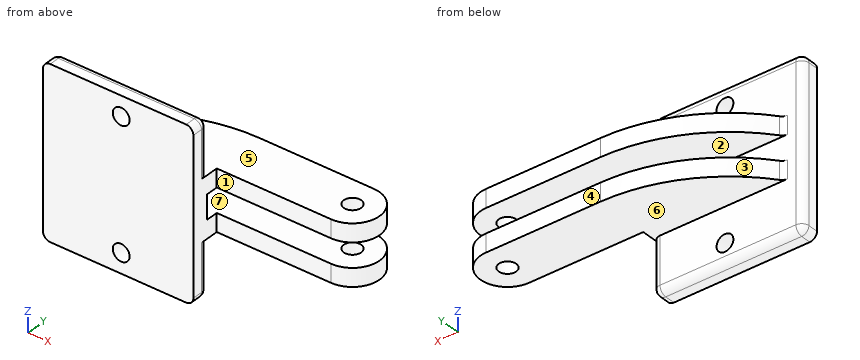
from build123d import *

# Parameters (mm, degrees)
SKETCH1_W           = 15.875
SKETCH1_H           = 17.78
SKETCH1_R           = 0.889
BOSS_EXTRUDE1_DEPTH = 1.8415
SKETCH2_R           = 0.92075
BOSS_EXTRUDE2_DEPTH = 3.175
SKETCH2_2_R         = 0.92075
CUT_EXTRUDE1_DEPTH  = 1.27
FILLET1_R           = 0.762


with BuildPart() as part:
    # Sketch1 → Boss-Extrude1 (new body)
    with BuildSketch(Plane(origin=(0, 0, 0), x_dir=(1, 0, 0), z_dir=(0, 1, 0))):
        Rectangle(SKETCH1_W, SKETCH1_H)
        with Locations((0.3175, 6.7945)):
            Circle(SKETCH1_R, mode=Mode.SUBTRACT)
        with Locations((0.3175, -6.7945)):
            Circle(SKETCH1_R, mode=Mode.SUBTRACT)
    extrude(amount=BOSS_EXTRUDE1_DEPTH)

    # Sketch2 → Boss-Extrude2 (add, symmetric)
    with BuildSketch(Plane.XY):
        with BuildLine():
            ThreePointArc((7.9375, 8.8265), (0.184776704, 6.981333441), (-5.9055, 1.8415))
            Line((-5.9055, 1.8415), (7.9375, 1.8415))
            Line((7.9375, 1.8415), (7.9375, 3.1115))
            Line((7.9375, 3.1115), (20.0025, 3.1115))
            ThreePointArc((20.0025, 3.1115), (22.86, 5.969), (20.0025, 8.8265))
            Line((20.0025, 8.8265), (7.9375, 8.8265))
        make_face()
        with Locations((20.0025, 5.969)):
            Circle(SKETCH2_R, mode=Mode.SUBTRACT)
    extrude(amount=BOSS_EXTRUDE2_DEPTH, both=True)

    # Sketch2<2> → Cut-Extrude1 (cut, symmetric)
    with BuildSketch(Plane.XY):
        with BuildLine():
            ThreePointArc((7.9375, 8.8265), (0.184776704, 6.981333441), (-5.9055, 1.8415))
            Line((-5.9055, 1.8415), (7.9375, 1.8415))
            Line((7.9375, 1.8415), (7.9375, 3.1115))
            Line((7.9375, 3.1115), (20.0025, 3.1115))
            ThreePointArc((20.0025, 3.1115), (22.86, 5.969), (20.0025, 8.8265))
            Line((20.0025, 8.8265), (7.9375, 8.8265))
        make_face()
        with Locations((20.0025, 5.969)):
            Circle(SKETCH2_2_R, mode=Mode.SUBTRACT)
    extrude(amount=CUT_EXTRUDE1_DEPTH, both=True, mode=Mode.SUBTRACT)

    # Fillet1
    fillet1_edges = [part.edges().sort_by_distance(p)[0] for p in [
        (7.9375, 1.8415, 6.0325),
        (0, 1.8415, -8.89),
        (7.9375, 1.8415, -6.0325),
        (-5.9055, 1.8415, 2.2225),
        (-5.9055, 1.8415, -2.2225),
        (-7.9375, 1.8415, 0),
        (-7.9375, 0.92075, -8.89),
        (7.9375, 0.92075, -8.89),
        (7.9375, 0.92075, 8.89),
        (-7.9375, 0.92075, 8.89),
        (0, 1.8415, 8.89),
    ]]
    fillet(fillet1_edges, radius=FILLET1_R)


solid = part.part
Verification items for the finished model (mm, model axes). Face numbers are marked on the shaded views. A direction names the side the tool comes from. Give positions to 0.01 mm unless a question says otherwise; leave off trailing zeros. Write each loop counter-clockwise with the first axis right and the second up, starting at its lowest first coordinate (ties: lowest second). Pieces come first, ordered by that corner, then holes. Notation, with made-up numbers: M -26.5,-20 L 6.5,-20 A22 cw 6.5,17 Z; hole C 27,80.5 d7. An arc over 180 degrees is marked long. Use CSV: the item, a comma, the result in double quotes.
1) Cross-section at C-C (z = -6.5). Enter the section's corners in (x, y).
Final values:
outline,"M -7.94,0 L -0.52,0 L -0.52,1.84 L -7.18,1.84 A0.76 ccw -7.94,1.08 Z; M 1.16,0 L 7.94,0 L 7.94,1.08 A0.76 ccw 7.18,1.84 L 1.16,1.84 Z"
2) Cross-section at D-D (z = 4.5). Enter the section's corners in (x, y), plus the area to 3 significant figures.
Final values:
outline,"M -7.94,0 L 7.94,0 L 7.94,1.08 A0.76 ccw 7.18,1.84 L -7.18,1.84 A0.76 ccw -7.94,1.08 Z"
area,"29.0 mm²"
3) Go/stop test with flat-tipped pins: pin 1 Ø2 at (x, z) = (0.32, 6.79) entering from +Y; pin 2 Ø7.5 at (x, z) = (1, 0.5) entering from +Y; pin 3 Ø2 at (x, y) = (-3.5, 5) entering from -Z (3 decimals). Record where each tip stops, or that it passes through.
Final values:
pin 1,"y = 1.84"
pin 2,"y = 8.51"
pin 3,"z = -3.175"
4) Access from +Z, -Z, +X, -X, +Y, -Y to the whole of each face (thin tool, end or side, straight path). Record for the marked faces 1, 2 and 3.
Final values:
face 1,"+Z, -Z, +X, -Y"
face 2,"+X, -X, +Y"
face 3,"+Z, -Z, -X, +Y"
5) Cross-section at A-A (x = 12.5). Enter the section's corners in (y, z) (1 decimal).
Final values:
outline,"M 3.1,-3.2 L 8.8,-3.2 L 8.8,-1.3 L 3.1,-1.3 Z; M 3.1,1.3 L 8.8,1.3 L 8.8,3.2 L 3.1,3.2 Z"
6) Material ranges on line 1 along Z through (x, y) = (18, 5.25) (3 decimals); line 2 along Y through (x, z) = (15, 2.5); line 3 along X through (y, z) = (0.5, 0.5), recorded low to high.
Final values:
line 1,"-3.175 to -1.27, 1.27 to 3.175"
line 2,"3.11 to 8.83"
line 3,"-7.94 to 7.94"
7) Cross-section at B-B (y = 4). Enter the section's corners in (x, z) (3 decimals), plus the area to 3 significant figures.
Final values:
outline,"M -4.014,-3.175 L 22.073,-3.175 L 22.073,-1.27 L -4.014,-1.27 Z; M -4.014,1.27 L 22.073,1.27 L 22.073,3.175 L -4.014,3.175 Z"
area,"99.4 mm²"
8) Release check for a two-part mould opening along Z. For the marked faces 4, 5, 6 and 7 record: released by +Z, released by -Z, zero draft, split by the parting line, or undercut.
Final values:
face 4,"zero draft"
face 5,"released by +Z"
face 6,"released by -Z"
face 7,"undercut"
